Source: CAD feature listing. Evaluate the final solid. Frame: model axes, mm. A direction names the side the tool comes from. Coordinates: 2 decimals unless noted, no trailing zeros. Order: outer loops, then holes, each group sorted by start corner. A loop starts at its lowest first (then second) coordinate and runs counter-clockwise, first axis right, second up. Notation, with made-up numbers: (1, 60.25) -> (45, 60.25) arc R15 ccw to (45, 88.25) -> close; hole circle Ø8 at (40.5, 23.25). An arc over 180 degrees is marked (long way). Write item = value, one per line. Start each with the question number.
Item 1: Mould query, pull axis Y, two halves, no side actions, for faces 1 (the flat face through (-3.85, 28.477, -6.794)), 2 (the flat face through (-7, 35.56, 4)), 3 (the flat face through (7, 16.51, 4)). Classes: released by +Y, released by -Y, zero draft, split by the parting line, or undercut.
Item 2: Set-up query: faces 4 (the flat face through (0, 2.54, -8)), 5 (the flat face through (0, 21.59, 8)), 6 (the flat face through (0, 35.56, 8)), 7 (the flat face through (7, 2.54, -4)). Return all of +Z, -Z, +X, -X, +Y, -Y with unobstructed straight access to the full face (end or side cutting, diameter ignored); none if empty.
Item 3: Contact query for a flat-ended pin moving along its axis: pin 1 (5 mm diameter, centred on x = 6, y = 22.5, fed in from -Z). Output: stop coordinate, or through.
Item 4: Section query D-D (z = -7.25). Output: boundary loops of the cut face in (x, y).
Item 5: Section query B-B (x = -5.75). Output: boundary loops of the cut face in (y, z), then the cut area to 3 significant figures.
Item 6: Ray query, line 1 along Y through (x, z) = (-6, 5.5); line 2 along X through (y, z) = (34, 0.25); line 3 along X through (y, z) = (8, 4). Return the intervals inside material, ascending. Write a range as [from, to].
Item 7: Section query A-A (y = 16). Output: boundary loops of the cut face in (x, z).
```python
from build123d import *

# Parameters (mm, degrees)
SKETCH1_R               = 6.35
BOSS_EXTRUDE1_DEPTH     = 38.1
CUT_EXTRUDE1_DEPTH      = 2.54
CUT_EXTRUDE2_START      = -2.54
CUT_EXTRUDE2_DEPTH      = 2.54
CUT_EXTRUDE3_DEPTH      = 2.54
CUT_EXTRUDE3_DEPTH_BACK = 2.54
SKETCH5_R               = 11.357347969
SKETCH5_R_2             = 7.808951066


with BuildPart() as part:
    # Sketch1 → Boss-Extrude1 (new body)
    with BuildSketch(Plane(origin=(0, 0, 0), x_dir=(1, 0, 0), z_dir=(0, 1, 0))):
        Polygon((0, 9.017), (-7.808951066, 4.5085), (-7.808951066, -4.5085), (0, -9.017), (7.808951066, -4.5085), (7.808951066, 4.5085), align=None)
        with Locations(Location((0, 0, 0), (0, 0, 90))):
            Circle(SKETCH1_R, mode=Mode.SUBTRACT)
    extrude(amount=BOSS_EXTRUDE1_DEPTH)

    # Sketch3 → Cut-Extrude1 (cut)
    with BuildSketch(Plane.XZ):
        with BuildLine():
            Line((7.808951066, -4.5085), (7.808951066, 0))
            ThreePointArc((7.808951066, 0), (6.762749987, -3.904475555), (3.904475488, -6.762750026))
            Line((3.904475488, -6.762750026), (7.808951066, -4.5085))
        make_face()
        with BuildLine():
            ThreePointArc((3.904475554, 6.762749988), (6.762750006, 3.904475522), (7.808951066, 0))
            Line((7.808951066, 0), (7.808951066, 4.5085))
            Line((7.808951066, 4.5085), (3.904475554, 6.762749988))
        make_face()
        with BuildLine():
            ThreePointArc((-3.904475468, 6.762750038), (5e-08, 7.808951066), (3.904475554, 6.762749988))
            Line((3.904475554, 6.762749988), (0, 9.017))
            Line((0, 9.017), (-3.904475468, 6.762750038))
        make_face()
        with BuildLine():
            Line((0, -9.017), (3.904475488, -6.762750026))
            ThreePointArc((3.904475488, -6.762750026), (-3.8e-08, -7.808951066), (-3.904475554, -6.762749988))
            Line((-3.904475554, -6.762749988), (0, -9.017))
        make_face()
        with BuildLine():
            ThreePointArc((-7.808951066, 1.5e-08), (-6.762749977, 3.904475572), (-3.904475468, 6.762750038))
            Line((-3.904475468, 6.762750038), (-7.808951066, 4.5085))
            Line((-7.808951066, 4.5085), (-7.808951066, 1.5e-08))
        make_face()
        with BuildLine():
            Line((-7.808951066, -4.5085), (-3.904475554, -6.762749988))
            ThreePointArc((-3.904475554, -6.762749988), (-6.76275001, -3.904475516), (-7.808951066, 1.5e-08))
            Line((-7.808951066, 1.5e-08), (-7.808951066, -4.5085))
        make_face()
    extrude(amount=-CUT_EXTRUDE1_DEPTH, mode=Mode.SUBTRACT)

    # Sketch4 → Cut-Extrude2 (cut)
    with BuildSketch(Plane(origin=(0, 38.1, 0), x_dir=(1, 0, 0), z_dir=(0, 1, 0)).offset(CUT_EXTRUDE2_START)):
        with BuildLine():
            Line((-7.808951066, -4.5085), (-3.904475554, -6.762749988))
            ThreePointArc((-3.904475554, -6.762749988), (-6.762750002, -3.904475529), (-7.808951066, -1.5e-08))
            Line((-7.808951066, -1.5e-08), (-7.808951066, -4.5085))
        make_face()
        with BuildLine():
            Line((0, -9.017), (3.904475554, -6.762749988))
            ThreePointArc((3.904475554, -6.762749988), (0, -7.808951066), (-3.904475554, -6.762749988))
            Line((-3.904475554, -6.762749988), (0, -9.017))
        make_face()
        with BuildLine():
            ThreePointArc((-7.808951066, -1.5e-08), (-6.76275001, 3.904475516), (-3.904475554, 6.762749988))
            Line((-3.904475554, 6.762749988), (-7.808951066, 4.5085))
            Line((-7.808951066, 4.5085), (-7.808951066, -1.5e-08))
        make_face()
        with BuildLine():
            ThreePointArc((-3.904475554, 6.762749988), (-5e-08, 7.808951066), (3.904475468, 6.762750038))
            Line((3.904475468, 6.762750038), (0, 9.017))
            Line((0, 9.017), (-3.904475554, 6.762749988))
        make_face()
        with BuildLine():
            ThreePointArc((3.904475468, 6.762750038), (6.762749981, 3.904475566), (7.808951066, 0))
            Line((7.808951066, 0), (7.808951066, 4.5085))
            Line((7.808951066, 4.5085), (3.904475468, 6.762750038))
        make_face()
        with BuildLine():
            Line((7.808951066, -4.5085), (7.808951066, 0))
            ThreePointArc((7.808951066, 0), (6.762750006, -3.904475522), (3.904475554, -6.762749988))
            Line((3.904475554, -6.762749988), (7.808951066, -4.5085))
        make_face()
    extrude(amount=CUT_EXTRUDE2_DEPTH, mode=Mode.SUBTRACT)

    # Sketch5 → Cut-Extrude3 (cut, two sides: drawn at the far end of the back side and taken through both)
    with BuildSketch(Plane(origin=(0, 19.05, 0), x_dir=(-1, 0, 0), z_dir=(0, -1, 0)).offset(-CUT_EXTRUDE3_DEPTH_BACK)):
        Circle(SKETCH5_R)
        with Locations(Location((0, 0, 0), (0, 0, 90))):
            Circle(SKETCH5_R_2, mode=Mode.SUBTRACT)
    extrude(amount=CUT_EXTRUDE3_DEPTH + CUT_EXTRUDE3_DEPTH_BACK, mode=Mode.SUBTRACT)


solid = part.part
```
Computed:
q1.face_1 = zero draft
q1.face_2 = released by +Y
q1.face_3 = undercut
q2.face_4 = -Z, -Y
q2.face_5 = +Z
q2.face_6 = +Z, +Y
q2.face_7 = -Z, +X, -Y
q3.pin_1 = -7
q4.outline = (-3.06, 2.54) -> (-2.9, 2.54) -> (-2.9, 0) -> (2.9, 0) -> (2.9, 2.54) -> (3.06, 2.54) -> (3.06, 16.51) -> (2.9, 16.51) -> (2.9, 21.59) -> (3.06, 21.59) -> (3.06, 35.56) -> (2.9, 35.56) -> (2.9, 38.1) -> (-2.9, 38.1) -> (-2.9, 35.56) -> (-3.06, 35.56) -> (-3.06, 21.59) -> (-2.9, 21.59) -> (-2.9, 16.51) -> (-3.06, 16.51) -> close
q5.outline = (0, -5.28) -> (2.54, -5.28) -> (2.54, -5.7) -> (16.51, -5.7) -> (16.51, -5.28) -> (21.59, -5.28) -> (21.59, -5.7) -> (35.56, -5.7) -> (35.56, -5.28) -> (38.1, -5.28) -> (38.1, -2.69) -> (0, -2.69) -> close; (0, 2.69) -> (38.1, 2.69) -> (38.1, 5.28) -> (35.56, 5.28) -> (35.56, 5.7) -> (21.59, 5.7) -> (21.59, 5.28) -> (16.51, 5.28) -> (16.51, 5.7) -> (2.54, 5.7) -> (2.54, 5.28) -> (0, 5.28) -> close
q5.area = 220 mm^2
q6.line_1 = [2.54, 16.51], [21.59, 35.56]
q6.line_2 = [-7.81, -6.35], [6.35, 7.81]
q6.line_3 = [-7.81, -4.93], [4.93, 7.81]
q7.outline = (-7.81, -4.51) -> (0, -9.02) -> (7.81, -4.51) -> (7.81, 4.51) -> (0, 9.02) -> (-7.81, 4.51) -> close; hole circle Ø12.7 at (0, 0)
